The drawing under review shows one solid part. Ordinate dimensions are in mm from its lowest x, y, z. A direction names the side the tool comes from. Give positions to 0.01 mm unless a question says otherwise; leave off trailing zeros. Loops run counter-clockwise (first coordinate to the right, second up) from the corner with the lowest first, then second, coordinate; pieces in that order, holes last. Notation, with made-up numbers: M 0,66 L 31,66 A15 cw 31,90 Z; hole C 3,61 d7. An arc over 180 degrees is marked long. One line per item, written item: value. Start each with the question number.
Q1. For the marked faces 1 and 2, list the 3-axis set-ups (+Z, -Z, +X, -X, +Y, -Y) from which the entire face can be reached by the end or side of a thin tool; tool diameter is ignored.
Q2. We need section C-C on z = 44. Write out the cut boundary in (x, y).
Q3. For pin 1 (1.5 mm diameter, centred on x = 84.5, y = 42, fed in from +Z); pin 2 (10 mm diameter, centred on x = 19, y = 33.5, fed in from +Z), all flat-tipped, find the tip position at first contact; note any pin that passes through.
Q4. To check wall thickness, follow line 1 along Z through (x, y) = (74, 69.5) (1 decimal); line 2 along Z through (x, y) = (80, 46); line 3 along X through (y, z) = (23.5, 36). State the ranges of each line that lie inside material, in increasing order. Write a range as from..to.
Q5. We need section D-D on x = 15.5. Write out the cut boundary in (y, z) (1 decimal).
Q6. We need section B-B on x = 61.5. Write out the cut boundary in (y, z) (1 decimal), plus the area to 3 significant figures.
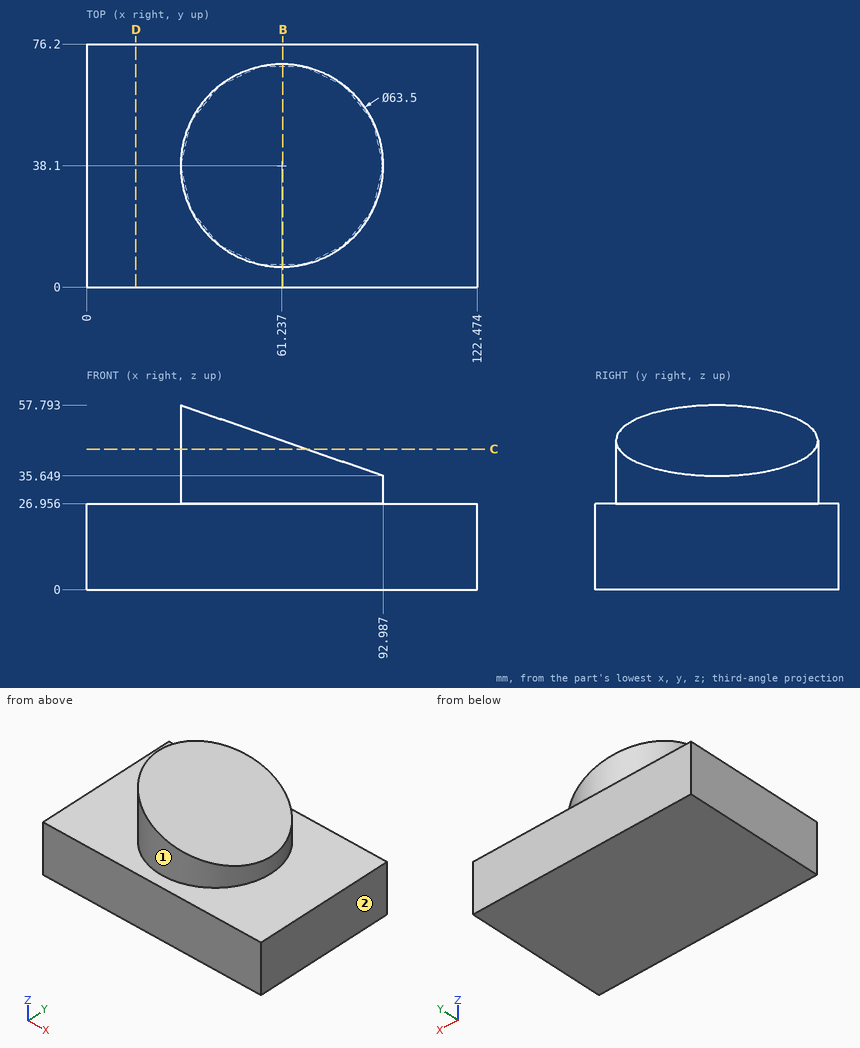
Solved:
1. face 1: +Z
1. face 2: +Z, -Z, +X, +Y, -Y
2. outline: M 69.04,7.32 L 69.04,68.88 A31.75 ccw long Z
3. pin 1: z = 38.87
3. pin 2: z = 26.96
4. line 1: 0..27
4. line 2: 0..40.18
4. line 3: 33.04..89.43
5. outline: M 0,0 L 76.2,0 L 76.2,27 L 0,27 Z
6. outline: M 0,0 L 76.2,0 L 76.2,27 L 69.8,27 L 69.8,46.6 L 6.4,46.6 L 6.4,27 L 0,27 Z
6. area: 3,300 mm2
